Work out the finished part from the listing and answer in its coordinate system (mm). A direction names the side the tool comes from. Coordinates: 2 decimals unless noted, no trailing zeros. Write each loop counter-clockwise with the first axis right and the second up, starting at its lowest first coordinate (ties: lowest second). Pieces come first, ordered by that corner, then holes. Notation, with made-up numbers: M 80,81.5 L 105,81.5 A22 ccw 105,94.5 Z; hole C 59,66 d2. An arc over 180 degrees is marked long. Use CSV: the item, a comma, the result in double quotes.
from build123d import *

# Parameters (mm, degrees)
SKETCH1_R           = 37.5
BOSS_EXTRUDE1_DEPTH = 35
SKETCH2_R           = 40
BOSS_EXTRUDE2_DEPTH = 10
SKETCH3_R           = 3
CUT_EXTRUDE1_DEPTH  = 10
CIRPATTERN1_COUNT   = 6


with BuildPart() as part:
    # Sketch1 → Boss-Extrude1 (new body)
    with BuildSketch(Plane(origin=(0, 0, 0), x_dir=(0, 0, -1), z_dir=(1, 0, 0))):
        Circle(SKETCH1_R)
    extrude(amount=BOSS_EXTRUDE1_DEPTH)

    # Sketch2 → Boss-Extrude2 (add)
    with BuildSketch(Plane(origin=(35, 0, 0), x_dir=(0, 0, -1), z_dir=(1, 0, 0))):
        Circle(SKETCH2_R)
    extrude(amount=BOSS_EXTRUDE2_DEPTH)

    # Sketch3 → Cut-Extrude1 (cut)
    with BuildSketch(Plane(origin=(0, 37.5, 0), x_dir=(1, 0, 0), z_dir=(0, 1, 0))):
        with Locations(Location((15, 0, 0), (0, 0, 270))):
            Circle(SKETCH3_R)
    cut_extrude1 = extrude(amount=-CUT_EXTRUDE1_DEPTH, mode=Mode.SUBTRACT)

    # CirPattern1: Cut-Extrude1 ×6 about axis
    cirpattern1_axis = Axis((0, 0, 0), (1, 0, 0))
    for i in range(1, CIRPATTERN1_COUNT):
        add(cut_extrude1.rotate(cirpattern1_axis, i * 360 / CIRPATTERN1_COUNT), mode=Mode.SUBTRACT)


solid = part.part
Item 1: Consider probe 1 along X at (y, z) = (34, 0); probe 2 along X at (y, z) = (-29, -2.5); probe 3 along Z at (x, y) = (15, -32.5). Determine where each line is inside the solid, lowest interval first.
Answer:
probe 1,"x = 0 to 12, 18 to 45"
probe 2,"x = 0 to 13.34, 16.66 to 45"
probe 3,"z = -18.71 to -3, 3 to 18.71"
Item 2: Given pin 1 (6 mm diameter, centred on x = 31, y = -10, fed in from +Z); pin 2 (3 mm diameter, centred on y = -24, z = 31, fed in from -X); pin 3 (2 mm diameter, centred on x = 12.5, z = 6.5, fed in from +Y), each flat-ended and moving along its own axis, determine where each tip first touches the part or whether it passes through.
Answer:
pin 1,"stops at z = 36.84"
pin 2,"stops at x = 35"
pin 3,"stops at y = 37.09"
Item 3: The part is cut by section A-A (y = 0). Write down the section's boundary in (x, z), then the cut area to 4 significant figures.
Answer:
outline,"M 0,-37.5 L 35,-37.5 L 35,-40 L 45,-40 L 45,40 L 35,40 L 35,37.5 L 0,37.5 Z"
area,"3,425 mm2"
Item 4: The part is cut by section C-C (x = 38). Write down the section's boundary in (y, z).
Answer:
outline,"C 0,0 d80"
Item 5: The part is cut by section D-D (y = -28.5). Write down the section's boundary in (x, z).
Answer:
outline,"M 0,-24.37 L 35,-24.37 L 35,-28.07 L 45,-28.07 L 45,28.07 L 35,28.07 L 35,24.37 L 0,24.37 Z; hole C 15,0 d6"
Item 6: The part is cut by section B-B (z = 0). Write down the section's boundary in (x, y), then the cut area to 4 significant figures.
Answer:
outline,"M 0,-37.5 L 12,-37.5 L 12,-27.5 L 18,-27.5 L 18,-37.5 L 35,-37.5 L 35,-40 L 45,-40 L 45,40 L 35,40 L 35,37.5 L 18,37.5 L 18,27.5 L 12,27.5 L 12,37.5 L 0,37.5 Z"
area,"3,305 mm2"
Item 7: For a pull along Y with two mould halves and no side action, classify faces 1 (the face through (45, 1, 1)), 2 (the face through (17.26, 37.18, 4.88)), 3 (the face through (15.04, 13.71, -23.84)) as released by +Y, released by -Y, zero draft, split by the parting line, or undercut.
Answer:
face 1,"zero draft"
face 2,"split by the parting line"
face 3,"undercut"
Item 8: A tool of negligible diameter and unlimited length cuts with its end or side. For faces 4 (the face through (15.042, 13.786, 23.795)), 5 (the face through (15, 27.5, 0)), 6 (the face through (12.07, -32.57, 0.65)), from which of +Z, -Z, +X, -X, +Y, -Y can it reach the whole face along a straight path? Write none if from no direction.
Answer:
face 4,"none"
face 5,"+Y"
face 6,"-Y"
